Autodesk Inventor part; units mm, degrees
ref_plane "YZ Plane" through (0, 0, 0) normal (1, 0, 0) x (0, 1, 0)
ref_plane "XZ Plane" through (0, 0, 0) normal (0, 1, 0) x (-1, 0, 0)
ref_plane "XY Plane" through (0, 0, 0) normal (0, 0, 1) x (1, 0, 0)
sketch "Szkic1" plane through (0, 0, 0) normal (0, 0, 1) x (1, 0, 0)
  line L0 (-6.9514, -9.6622) -> (35.0486, -9.6622)
  line L1 (35.0486, -9.6622) -> (35.0486, 7.8378)
  line L2 (35.0486, 7.8378) -> (-6.9514, 7.8378)
  line L3 (-6.9514, 7.8378) -> (-6.9514, -9.6622)
  point P0 (0, 0)
  point P1 (-1.2014, -4.6622)
  point P2 (29.2986, -4.6622)
  dimension "d0" = 42
  dimension "d1" = 17.5
  dimension "d2" = 5.75
  dimension "d3" = 5
  dimension "d4" = 5
  dimension "d5" = 5.75
extrude "Wyciągnięcie proste1" add sketch "Szkic1" along normal blind 20
hole "Otwór1" at (-1.2014, -4.6622, 0) at (29.2986, -4.6622, 0) direction (0, 0, 1) diameter 5 end through all
sketch "Szkic2" plane through (-6.9514, -9.6622, 0) normal (0, -1, 0) x (1, 0, 0)
  line L0 (0, 0) -> (42, 0)
  line L1 (42, 0) -> (42, 20)
  line L2 (0, 20) -> (42, 20)
  line L3 (0, 0) -> (0, 20)
  circle A0 centre (21, 10) radius 5.025
  line L4 (23.9012, 15.025) -> (26.8024, 10)
  line L5 (26.8024, 10) -> (23.9012, 4.975)
  line L6 (23.9012, 4.975) -> (18.0988, 4.975)
  line L7 (18.0988, 4.975) -> (15.1976, 10)
  line L8 (15.1976, 10) -> (18.0988, 15.025)
  line L9 (18.0988, 15.025) -> (23.9012, 15.025)
  circle A1 centre (21, 10) radius 3.25
  point P0 (6.9514, 0)
  point P1 (21, 15.025)
  dimension "d19" = 10.05
  dimension "d15" = 42
  dimension "d16" = 20
  dimension "d17" = 10
  dimension "d18" = 21
  dimension "d20" = 6.5
extrude "Wyciągnięcie proste2" cut sketch "Szkic2" against normal through all contours A1
extrude "Wyciągnięcie proste3" cut sketch "Szkic2" against normal blind 10 contours A0 | A0 L4 L5 | A0 L9 L4 | L5 L6 A0 | A0 L8 L9 | L6 L7 A0 | A0 L7 L8
chamfer "Faza1" distance 0.6 angle 45 1 edges at (10.7986, 7.8378, 10)
fillet "Zaokrąglenie1" radius 1 2 edges at (-6.9514, -9.6622, 10) (35.0486, -9.6622, 10)
chamfer "Faza2" distance 2 angle 45 2 edges at (-6.9514, 7.8378, 10) (35.0486, 7.8378, 10)
properties part number "3DP_ABS_Z_Axis_Screw_Nut_Mount"
Check sheet for the modelled part. Datum: model origin and axes. Units: mm. A direction names the side the tool comes from. Round coordinates to 2 decimals unless told otherwise and drop trailing zeros. Order: outer loops, then holes, each group sorted by start corner. A loop starts at its lowest first (then second) coordinate and runs counter-clockwise, first axis right, second up. Notation, with made-up numbers: M 87,58.5 L 133,58.5 A17 ccw 133,79.5 Z; hole C 30,67 d2. An arc over 180 degrees is marked long. Answer in a Markdown table with one row per item.
(1) Section check A-A on y = 4.75. Record the boundary of the cut face in (x, z), plus the area to 3 significant figures.
Findings:
| item | result |
|---|---|
| outline | M -6.95,0 L 35.05,0 L 35.05,20 L -6.95,20 Z; hole C 14.05,10 d6.5 |
| area | 807 mm^2 |
(2) Section check D-D on z = 17.5. Record the boundary of the cut face in (x, y).
Findings:
| item | result |
|---|---|
| outline | M -6.95,-8.66 A1 ccw -5.95,-9.66 L 34.05,-9.66 A1 ccw 35.05,-8.66 L 35.05,5.84 L 33.05,7.84 L -4.95,7.84 L -6.95,5.84 Z; hole C -1.2,-4.66 d5; hole C 29.3,-4.66 d5 |
(3) Draft check along X on faces 1 (the cylindrical face through (27.2, -3.3, 10.1)), 2 (the flat face through (-5.97, 6.82, 10.14)), 3 (the flat face through (19, 7.838, 10)). Enter one of: +X half, -X half, draft (parallel to the pull), parting line (faces both ways), or undercut.
Findings:
| item | result |
|---|---|
| face 1 | undercut |
| face 2 | -X half |
| face 3 | draft |
(4) Set-up check for faces 4 (the flat face through (14, -5, 15.025)), 5 (the flat face through (-6.951, -1, 10)): record each of +Z, -Z, +X, -X, +Y, -Y from which the full face is reachable in a straight line by a thin tool's end or side.
Findings:
| item | result |
|---|---|
| face 4 | -Y |
| face 5 | +Z, -Z, -X, +Y, -Y |
(5) Gauge pin test, flat ends, axial feed: pin 1 (5 mm diameter, centred on x = 12.5, z = 9, fed in from -Y); pin 2 (6 mm diameter, centred on x = -1.2, y = -4.66, fed in from +Z); pin 3 (3 mm diameter, centred on x = 29.3, y = -4.66, fed in from -Z); pin 4 (5 mm diameter, centred on x = 14, z = 9, fed in from +Y). Record the tip position at first contact, or that the pin passes through.
Findings:
| item | result |
|---|---|
| pin 1 | stops at y = 0.34 |
| pin 2 | stops at z = 20 |
| pin 3 | passes through |
| pin 4 | stops at y = 7.49 |
(6) Section check C-C on y = -6.75. Record the boundary of the cut face in (x, z) (3 decimals), plus the area to 3 significant figures.
Findings:
| item | result |
|---|---|
| outline | M -6.951,0 L -2.577,0 L -2.577,20 L -6.951,20 Z; M 0.174,0 L 27.923,0 L 27.923,20 L 0.174,20 Z; M 30.674,0 L 35.049,0 L 35.049,20 L 30.674,20 Z; hole M 8.246,10 L 11.147,4.975 L 16.95,4.975 L 19.851,10 L 16.95,15.025 L 11.147,15.025 Z |
| area | 643 mm^2 |
(7) Section check B-B on x = -3. Record the boundary of the cut face in (y, z).
Findings:
| item | result |
|---|---|
| outline | M -9.66,0 L -6.4,0 L -6.4,20 L -9.66,20 Z; M -2.93,0 L 7.84,0 L 7.84,20 L -2.93,20 Z |
(8) Material ranges on line 1 along X through (y, z) = (-5, 19); line 2 along X through (y, z) = (-4, 12); line 3 along X through (y, z) = (-3.75, 7.5), recorded low to high. Write a range as from..to.
Findings:
| item | result |
|---|---|
| line 1 | x = -6.95..-3.68, 1.28..26.82, 31.78..35.05 |
| line 2 | x = -6.95..-3.61, 1.21..9.4, 18.7..26.89, 31.71..35.05 |
| line 3 | x = -6.95..-3.53, 1.13..9.69, 18.41..26.97, 31.63..35.05 |
